from build123d import *

# Parameters (mm, degrees)
SKETCH1_R           = 53
SKETCH1_R_2         = 45
BOSS_EXTRUDE1_DEPTH = 14
SKETCH2_R           = 2.4
CUT_EXTRUDE1_DEPTH  = 4
SKETCH3_R           = 1.6
CUT_EXTRUDE2_DEPTH  = 6


with BuildPart() as part:
    # Sketch1 → Boss-Extrude1 (new body)
    with BuildSketch(Plane(origin=(0, 0, 0), x_dir=(1, 0, 0), z_dir=(0, 1, 0))):
        with Locations(Location((0, 0, 0), (0, 0, 270))):
            Circle(SKETCH1_R)
        with Locations(Location((0, 0, 0), (0, 0, 270))):
            Circle(SKETCH1_R_2, mode=Mode.SUBTRACT)
    extrude(amount=BOSS_EXTRUDE1_DEPTH)

    # Sketch2 → Cut-Extrude1 (cut)
    with BuildSketch(Plane.XZ):
        with Locations(Location((0, 49, 0), (0, 0, 270))):
            Circle(SKETCH2_R)
        with Locations(Location((42.435244785, 24.5, 0), (0, 0, 270))):
            Circle(SKETCH2_R)
        with Locations(Location((42.435244785, -24.5, 0), (0, 0, 270))):
            Circle(SKETCH2_R)
        with Locations(Location((0, -49, 0), (0, 0, 270))):
            Circle(SKETCH2_R)
        with Locations(Location((-42.435244785, -24.5, 0), (0, 0, 270))):
            Circle(SKETCH2_R)
        with Locations(Location((-42.435244785, 24.5, 0), (0, 0, 270))):
            Circle(SKETCH2_R)
    extrude(amount=-CUT_EXTRUDE1_DEPTH, mode=Mode.SUBTRACT)

    # Sketch3 → Cut-Extrude2 (cut)
    with BuildSketch(Plane.XZ):
        with Locations(Location((0, 49, 0), (0, 0, 270))):
            Circle(SKETCH3_R)
        with Locations(Location((42.435244785, 24.5, 0), (0, 0, 270))):
            Circle(SKETCH3_R)
        with Locations(Location((42.435244785, -24.5, 0), (0, 0, 270))):
            Circle(SKETCH3_R)
        with Locations(Location((0, -49, 0), (0, 0, 270))):
            Circle(SKETCH3_R)
        with Locations(Location((-42.435244785, 24.5, 0), (0, 0, 270))):
            Circle(SKETCH3_R)
        with Locations(Location((-42.435244785, -24.5, 0), (0, 0, 270))):
            Circle(SKETCH3_R)
    extrude(amount=-CUT_EXTRUDE2_DEPTH, mode=Mode.SUBTRACT)


solid = part.part
Geometry: final body of the model. Coordinates: model frame, mm. A direction names the side the tool comes from. Give positions to 0.01 mm unless a question says otherwise; leave off trailing zeros. Order: outer loops, then holes, each group sorted by start corner. A loop starts at its lowest first (then second) coordinate and runs counter-clockwise, first axis right, second up. Notation, with made-up numbers: (9.25, -30) -> (45.25, -30) arc R9 ccw to (45.25, -14) -> close; hole circle Ø7 at (59.5, -29.5). An arc over 180 degrees is marked (long way). Put each result on its own line as item: value.
Q1. Section C-C, the plane y = 11.75. Return loops of the section in (x, z).
Here are the results:
outline: circle Ø106 at (0, 0); hole circle Ø90 at (0, 0)
Q2. Pin query (flat end, axial travel): pin 1 (1.4 mm diameter, centred on x = -42, z = 24.5, fed in from -Y); pin 2 (2 mm diameter, centred on x = -39.5, y = 1.5, fed in from -Z); pin 3 (6 mm diameter, centred on y = 2.5, z = -2, fed in from +X). Return the tip coordinate at first contact, or that it passes through.
Here are the results:
pin 1: stops at y = 6
pin 2: stops at z = -36.42
pin 3: stops at x = 53
Q3. Section D-D, the plane x = 32.5. Return loops of the section in (y, z), then the cut area to 3 significant figures.
Here are the results:
outline: (0, -41.87) -> (14, -41.87) -> (14, -31.12) -> (0, -31.12) -> close; (0, 31.12) -> (14, 31.12) -> (14, 41.87) -> (0, 41.87) -> close
area: 301 mm^2
Q4. Section A-A, the plane x = 0. Return loops of the section in (y, z), then the cut area to 3 significant figures.
Here are the results:
outline: (0, -53) -> (14, -53) -> (14, -45) -> (0, -45) -> (0, -46.6) -> (4, -46.6) -> (4, -47.4) -> (6, -47.4) -> (6, -50.6) -> (4, -50.6) -> (4, -51.4) -> (0, -51.4) -> close; (0, 45) -> (14, 45) -> (14, 53) -> (0, 53) -> (0, 51.4) -> (4, 51.4) -> (4, 50.6) -> (6, 50.6) -> (6, 47.4) -> (4, 47.4) -> (4, 46.6) -> (0, 46.6) -> close
area: 173 mm^2
Q5. Draft query along X for faces 3 (the face through (52.55, 6.9, -6.9)), 4 (the face through (-39, 14, -24)), 5 (the face through (40.97, 1.97, 26.4)), 6 (the face through (-2, 4, -49)). Return one class per face: released by +X, released by -X, zero draft, split by the parting line, or undercut.
Here are the results:
face 3: split by the parting line
face 4: zero draft
face 5: undercut
face 6: undercut
Q6. Reachability of faces 1 (the face through (-17.235, 6.902, 41.569)), 2 (the face through (-40.85, 4.99, -24.29)) from +Z, -Z, +X, -X, +Y, -Y: full face, straight path, thin tool, end or side. Return the list, or none.
Here are the results:
face 1: +Y, -Y
face 2: -Y
Q7. Material intervals for L1, parallel to X at y = 4.5, z = -24.5; L2, parallel to X at y = 5.25, z = 0; L3, parallel to X at y = 1, z = 24.5, sorted ascending.
Here are the results:
L1: x = -47 to -44.04, -40.84 to -37.75, 37.75 to 40.84, 44.04 to 47
L2: x = -53 to -45, 45 to 53
L3: x = -47 to -44.84, -40.04 to -37.75, 37.75 to 40.04, 44.84 to 47
Q8. Section B-B, the plane z = 0. Return loops of the section in (x, y), then the cut area to 3 significant figures.
Here are the results:
outline: (-53, 0) -> (-45, 0) -> (-45, 14) -> (-53, 14) -> close; (45, 0) -> (53, 0) -> (53, 14) -> (45, 14) -> close
area: 224 mm^2
